```python
from build123d import *

# Parameters (mm, degrees)
SKETCH1_R           = 30
BOSS_EXTRUDE1_DEPTH = 30
FILLET1_R           = 15
SKETCH2_R           = 2.5
CUT_EXTRUDE1_DEPTH  = 52.961524227


with BuildPart() as part:
    # Sketch1 → Boss-Extrude1 (new body)
    with BuildSketch(Plane.XY):
        Circle(SKETCH1_R)
    extrude(amount=BOSS_EXTRUDE1_DEPTH)

    # Fillet1
    fillet1_edges = [part.edges().sort_by_distance(p)[0] for p in [
        (-30, 0, 0),
        (-30, 0, 30),
    ]]
    fillet(fillet1_edges, radius=FILLET1_R - 0.0001)  # a hair under: the kernel refuses the full size

    # Sketch2 → Cut-Extrude1 (cut, through all)
    with BuildSketch(Plane(origin=(0, 0, 0), x_dir=(-1, 0, 0), z_dir=(0, 0, -1))):
        Circle(SKETCH2_R)
    extrude(amount=-CUT_EXTRUDE1_DEPTH, mode=Mode.SUBTRACT)


solid = part.part
```
Geometry check sheet. Reference: the model listing, model coordinates, mm. Give positions to 0.01 mm unless a question says otherwise; leave off trailing zeros. Write each loop counter-clockwise with the first axis right and the second up, starting at its lowest first coordinate (ties: lowest second). Pieces come first, ordered by that corner, then holes.
1) Section check C-C, the plane z = 14. Record the boundary of the cut face in (x, y), and give its area (3 significant figures).
2) Material ranges on L1, parallel to Z at x = -24, y = -7; L2, parallel to Y at x = 19, z = 15; L3, parallel to Y at x = -19.5, z = 23.5, recorded low to high.
3) Gauge pin test, flat ends, axial feed: pin 1 (12 mm diameter, centred on x = -18, y = 7, fed in from -Z); pin 2 (8 mm diameter, centred on x = -22.5, z = 9, fed in from +Y); pin 3 (1 mm diameter, centred on x = 13.5, y = -23.5, fed in from +Z); pin 4 (1 mm diameter, centred on y = -11.5, z = 16.5, fed in from -X). Record the tip position at first contact, or that the pin passes through.
4) Section check D-D, the plane z = 18. Record the boundary of the cut face in (x, y).
5) Release check for a two-part mould opening along Y. For faces 1 (the flat face through (0, -3, 0)), 2 (the cylindrical face through (0.54, -2.44, 14.79)) record: pulls with the +Y half, pulls with the -Y half, needs draft (parallel to the pull), parting line crosses it, or undercut.
Computed:
1. outline: circle Ø59.93 at (0, 0); hole circle Ø5 at (0, 0)
1. area: 2,800 mm2
2. L1: z = 3.82 to 26.18
2. L2: y = -23.22 to 23.22
2. L3: y = -19.19 to 19.19
3. pin 1: stops at z = 0
3. pin 2: stops at y = 22.5
3. pin 3: stops at z = 24.51
3. pin 4: stops at x = -27.84
4. outline: circle Ø59.39 at (0, 0); hole circle Ø5 at (0, 0)
5. face 1: needs draft
5. face 2: undercut
